Source: CAD feature listing. Evaluate the final solid. Frame: model axes, mm. A direction names the side the tool comes from. Give positions to 0.01 mm unless a question says otherwise; leave off trailing zeros. Loops run counter-clockwise (first coordinate to the right, second up) from the corner with the lowest first, then second, coordinate; pieces in that order, holes last. Notation, with made-up numbers: (16.25, -19.75) -> (52.25, -19.75) arc R17 cw to (52.25, 5.25) -> close; hole circle Ø8 at (12.25, -21). An arc over 180 degrees is marked (long way). Return JSON: item names as keys, results as strings. Group by question number.
(1) Ray query, line 1 (Z direction, x = 0, y = 85.15) (3 decimals); line 2 (Z direction, x = 0, y = 87.5) (3 decimals); line 3 (Y direction, x = 0, z = 28.7) (3 decimals). Return the intervals inside material, ascending. Write a range as from..to.
(2) Cut plane A-A on y = 74.7. Return loops of the section in (x, z), then the cut area to 3 significant figures.
(3) Draft query along Y for faces 1 (the face through (0.5, 61, 11)), 2 (the face through (0, 82, 13)), 3 (the face through (0, 63, 27.5)), 4 (the face through (4.5, 48, 17)). Return one class per face: released by +Y, released by -Y, zero draft, split by the parting line, or undercut.
(4) Cut plane C-C on z = 30.5. Return loops of the section in (x, y) (3 decimals), then the cut area to 3 significant figures.
(5) Cut plane D-D on y = 63. Return loops of the section in (x, z), then the cut area to 3 significant figures.
(6) Access query for faces 5 (the face through (0, 82, 21)), 6 (the face through (2.528, 64.794, 8.081)), 7 (the face through (-0.11, 6.764, 10.873)). Directions: +Z, -Z, +X, -X, +Y, -Y. A direction counts if a zero-diameter tool reaches every point of the face in a straight line with its end or side. Return the directions, or none.
(7) Cut plane B-B on z = 8. Return loops of the section in (x, y) (3 decimals), then the cut area to 3 significant figures.
(8) Pin query (flat end, axial travel): pin 1 (1.4 mm diameter, centred on x = 0, z = 12, fed in from +Y); pin 2 (3 mm diameter, centred on x = -0.5, z = 8, fed in from -Y); pin 3 (4 mm diameter, centred on x = -1, y = 41, fed in from -Z); pin 4 (2 mm diameter, centred on x = -0.5, y = 64, fed in from +Z). Return the tip coordinate at first contact, or that it passes through.
Autodesk Inventor part; units mm, degrees
ref_plane "Work Plane2" through (-89, -40.3889, 33.5) normal (0, 0, 1) x (1, 0, 0)
ref_plane "YZ Plane" through (0, 0, 0) normal (1, 0, 0) x (0, 1, 0)
ref_plane "XZ Plane" through (0, 0, 0) normal (0, 1, 0) x (-1, 0, 0)
ref_plane "Work Plane1" through (0, 0, 0) normal (0, 0, 1) x (1, 0, 0)
ref_plane "Work Plane2" through (-89, -40.3889, 33.5) normal (0, 0, 1) x (1, 0, 0)
sketch "Sketch1" plane through (0, 0, 0) normal (0, 0, 1) x (1, 0, 0)
  line L0 (23.5, 88.5) -> (-23.5, 88.5)
  line L1 (-23.5, 88.5) -> (-23.5, 36.5)
  line L2 (-26.5, 33.5) -> (-89, 33.5)
  line L3 (-89, 33.5) -> (-89, -72.5)
  line L4 (-89, -72.5) -> (-77, -72.5)
  line L5 (-74, -75.5) -> (-74, -93.5)
  line L6 (-74, -93.5) -> (74, -93.5)
  line L7 (74, -93.5) -> (74, -75.5)
  line L8 (77, -72.5) -> (89, -72.5)
  line L9 (89, -72.5) -> (89, 33.5)
  line L10 (89, 33.5) -> (26.5, 33.5)
  line L11 (23.5, 36.5) -> (23.5, 88.5)
  line L12 (-4.5, 81.5) -> (-4.5, 36.5)
  line L13 (-7.5, 33.5) -> (-13.5, 33.5)
  line L14 (-16.5, 36.5) -> (-16.5, 81.5)
  line L15 (7.5, 84.5) -> (13.5, 84.5)
  line L16 (16.5, 81.5) -> (16.5, 36.5)
  line L17 (13.5, 33.5) -> (7.5, 33.5)
  line L18 (4.5, 36.5) -> (4.5, 81.5)
  line L19 (-13.5, 84.5) -> (-7.5, 84.5)
  line L20 (-4.5, 88.5) -> (4.5, 88.5)
  line L21 (4.5, 88.5) -> (4.5, 5.75)
  line L22 (4.5, 5.75) -> (-4.5, 5.75)
  line L23 (-4.5, 5.75) -> (-4.5, 88.5)
  line L24 (-32.2, 4.75) -> (-59.9, 4.75)
  arc A0 (13.5, 33.5) -> (16.5, 36.5) centre (13.5, 36.5) ccw
  arc A1 (4.5, 36.5) -> (7.5, 33.5) centre (7.5, 36.5) ccw
  arc A2 (7.5, 84.5) -> (4.5, 81.5) centre (7.5, 81.5) ccw
  arc A3 (16.5, 81.5) -> (13.5, 84.5) centre (13.5, 81.5) ccw
  arc A4 (-4.5, 81.5) -> (-7.5, 84.5) centre (-7.5, 81.5) ccw
  arc A5 (-7.5, 33.5) -> (-4.5, 36.5) centre (-7.5, 36.5) ccw
  arc A6 (-16.5, 36.5) -> (-13.5, 33.5) centre (-13.5, 36.5) ccw
  arc A7 (-13.5, 84.5) -> (-16.5, 81.5) centre (-13.5, 81.5) ccw
  arc A8 (-26.5, 33.5) -> (-23.5, 36.5) centre (-26.5, 36.5) ccw
  arc A9 (-74, -75.5) -> (-77, -72.5) centre (-77, -75.5) ccw
  arc A10 (77, -72.5) -> (74, -75.5) centre (77, -75.5) ccw
  arc A11 (23.5, 36.5) -> (26.5, 33.5) centre (26.5, 36.5) ccw
  circle A12 centre (21.5, -85.5) radius 1.8
  circle A13 centre (-64.5, -85.5) radius 1.8
  circle A14 centre (83.4, -16.3889) radius 1.8
  circle A15 centre (-83.4, -19.2889) radius 1.8
  circle A16 centre (-21.5, -85.5) radius 1.8
  circle A17 centre (64.5, -85.5) radius 1.8
  circle A18 centre (-56.0375, 15.0937) radius 1.0065
  circle A19 centre (39.125, 4.3375) radius 1.0065
  circle A20 centre (-72.95, 4.275) radius 1.0065
  circle A21 centre (39.125, 25.9125) radius 1.0065
  circle A22 centre (72.95, 12.275) radius 1.0065
  circle A23 centre (86, 30.5) radius 1.0065
  circle A24 centre (-86, 30.5) radius 1.0065
  circle A25 centre (-39.125, 12.3375) radius 1.0065
  circle A26 centre (-72.95, 25.975) radius 1.0065
  circle A27 centre (-72.95, 12.275) radius 1.0065
  circle A28 centre (-39.125, 25.9125) radius 1.0065
  circle A29 centre (-86, 7.75) radius 1.0065
  circle A30 centre (86, 7.75) radius 1.0065
  circle A31 centre (72.95, 25.975) radius 1.0065
  circle A32 centre (39.125, 12.3375) radius 1.0065
  circle A33 centre (-39.125, 4.3375) radius 1.0065
  circle A34 centre (72.95, 4.275) radius 1.0065
  circle A35 centre (56.0375, 15.125) radius 1.0065
  circle A36 centre (78, -67.1725) radius 1.2295
  circle A37 centre (-24.1, -73.1) radius 1.2295
  circle A38 centre (24.1, -24.9) radius 1.2295
  circle A39 centre (-42.5, -43.2802) radius 1.2295
  circle A40 centre (-79, -42.3889) radius 1.2295
  circle A41 centre (-19.5, 28.875) radius 1.2295
  circle A42 centre (19.5, 9.55) radius 1.2295
  circle A43 centre (19.5, 47.3) radius 1.2295
  circle A44 centre (-19.5, 47.3) radius 1.2295
  circle A45 centre (0, 74.7) radius 1.2295
  circle A46 centre (-19.4231, 74.8077) radius 1.2295
  circle A47 centre (19.5, 74.7) radius 1.2295
  circle A48 centre (0, 49.05) radius 1.2295
  circle A49 centre (19.5, 28.875) radius 1.2295
  circle A50 centre (0, 19.125) radius 1.2295
  circle A51 centre (-19.5, 9.55) radius 1.2295
  circle A52 centre (-78, -67.1725) radius 1.2295
  circle A53 centre (-24.1, -24.9) radius 1.2295
  circle A54 centre (24.1, -73.1) radius 1.2295
  circle A55 centre (42.5, -42.7745) radius 1.2295
  circle A56 centre (79, -42.3889) radius 1.2295
  point P0 (0, 0)
  point P1 (-4.5, 81.5)
  point P2 (-4.5, 36.5)
  point P3 (7.5, 81.5)
  point P4 (13.5, 81.5)
  point P5 (-7.5, 81.5)
  point P6 (-13.5, 81.5)
  dimension "d41" = 1
extrude "Extrusion1" add sketch "Sketch1" along normal up to surface (33.5 mm away) contours L21 L18 L22 L23 L12 L0 | A45 | A48 | A50
sketch "Sketch2" plane through (4.5, 5.75, 0) normal (1, 0, 0) x (0, 0, -1)
  circle A0 centre (-23.4363, 28.1825) radius 2
  point P0 (0, -5.75)
extrude "Extrusion2" cut sketch "Sketch2" against normal blind 10
sketch "Sketch3" plane through (4.5, 5.75, 0) normal (1, 0, 0) x (0, 0, -1)
  circle A0 centre (-10.5, 55.25) radius 4.5
  point P0 (0, -5.75)
extrude "Extrusion3" cut sketch "Sketch3" against normal blind 4
sketch "Sketch4" plane through (-4.5, 5.75, 0) normal (-1, 0, 0) x (0, 0, 1)
  circle A0 centre (10.5, 55.25) radius 4.5
  point P0 (0, -5.75)
extrude "Extrusion4" cut sketch "Sketch4" against normal blind 4
sketch "Sketch5" plane through (-4.5, 5.75, 33.5) normal (0, 0, 1) x (1, 0, 0)
  line L0 (5, 59.75) -> (5, 50.75)
  line L1 (4, 50.75) -> (4, 59.75)
  line L2 (9, 26.1825) -> (0, 26.1825)
  line L3 (9, 30.1825) -> (0, 30.1825)
  line L4 (17, 78.15) -> (-8, 78.15)
  line L5 (-8, 35.85) -> (17, 35.85)
  line L6 (9, 82.75) -> (9, 0)
  line L7 (0, 50.75) -> (0, 59.75)
  line L8 (9, 35.85) -> (0, 35.85)
  line L9 (0, 35.85) -> (0, 50.75)
  line L10 (0, 50.75) -> (9, 50.75)
  line L11 (9, 50.75) -> (9, 35.85)
  line L12 (0, 0) -> (0, 82.75)
  line L13 (9, 78.15) -> (0, 78.15)
  line L14 (0, 78.15) -> (0, 59.75)
  line L15 (0, 59.75) -> (9, 59.75)
  line L16 (9, 59.75) -> (9, 78.15)
  line L17 (-18, 6.625) -> (-18, 20.125)
  line L18 (-18, 13.375) -> (27, 13.375)
  line L19 (9, 35.85) -> (0, 50.75)
  line L20 (9, 59.75) -> (9, 50.75)
  line L21 (0, 35.85) -> (9, 50.75)
  line L22 (9, 59.75) -> (0, 78.15)
  line L23 (0, 59.75) -> (9, 78.15)
  point P0 (4.5, -5.75)
  point P1 (4.5, 13.375)
  point P2 (4.5, 43.3)
  point P3 (4.5, 68.95)
  dimension "d9" = 4.5
  dimension "d10" = 4.5
hole "Hole1" at (0, 19.125, 33.5) at (0, 49.05, 33.5) at (0, 74.7, 33.5) direction (0, 0, -1) diameter 3.6 end through all countersink diameter 6.6 countersink angle 90
sketch "Sketch6" plane through (-4.5, 5.75, 0) normal (0, -1, 0) x (1, 0, 0)
  line L0 (9, 33.5) -> (0, 33.5)
  line L1 (0, 0) -> (0, 33.5)
  line L2 (0, 0) -> (9, 0)
  line L3 (9, 0) -> (9, 33.5)
  line L4 (0, 16.75) -> (9, 16.75)
  line L5 (9, 16.75) -> (0, 33.5)
  line L6 (9, 33.5) -> (0, 16.75)
  line L7 (0, 16.75) -> (9, 0)
  line L8 (9, 16.75) -> (0, 0)
  point P0 (4.5, 0)
  point P1 (4.5, 8.375)
  point P2 (4.5, 25.125)
hole "Hole2" at (0, 5.75, 8.375) at (0, 5.75, 25.125) direction (0, 1, 0) diameter 4 depth 6.6 counterbore diameter 5 counterbore depth 2
sketch "Sketch7" plane through (-4.5, 88.5, 0) normal (0, 1, 0) x (1, 0, 0)
  line L0 (0, -33.5) -> (9, -33.5)
  line L1 (0, -33.5) -> (9, -33.5)
  line L2 (9, 0) -> (9, -33.5)
  line L3 (9, 0) -> (0, 0)
  line L4 (0, 0) -> (0, -33.5)
  line L5 (-8, -1.4) -> (-8, -6.6)
  line L6 (-8, -32.1) -> (-8, -26.9)
  line L7 (17, -32.1) -> (17, -26.9)
  line L8 (17, -1.4) -> (17, -6.6)
  line L9 (17, -32.1) -> (-8, -32.1)
  line L10 (-8, -32.1) -> (-8, -26.9)
  line L11 (-8, -26.9) -> (17, -26.9)
  line L12 (17, -26.9) -> (17, -32.1)
  line L13 (-8, -6.6) -> (17, -6.6)
  line L14 (17, -6.6) -> (17, -1.4)
  line L15 (17, -1.4) -> (-8, -1.4)
  line L16 (-8, -1.4) -> (-8, -6.6)
  line L17 (17, -6.6) -> (-8, -6.6)
  line L18 (-8, -6.6) -> (-8, -8.6)
  line L19 (-8, -8.6) -> (17, -8.6)
  line L20 (17, -8.6) -> (17, -6.6)
  line L21 (-8, -26.9) -> (17, -26.9)
  line L22 (17, -26.9) -> (17, -24.9)
  line L23 (17, -24.9) -> (-8, -24.9)
  line L24 (-8, -24.9) -> (-8, -26.9)
  line L25 (9, 0) -> (9, -33.5)
  line L26 (9, -16.75) -> (0, -16.75)
  line L27 (0, 0) -> (0, -33.5)
  line L28 (9, -24.9) -> (0, -16.75)
  line L29 (9, -8.6) -> (0, -16.75)
  line L30 (0, -8.6) -> (9, -16.75)
  line L31 (9, -16.75) -> (0, -24.9)
  point P0 (4.5, 0)
  point P1 (4.5, -20.825)
  point P2 (4.5, -12.675)
  dimension "d25" = 2
  dimension "d26" = 2
hole "Hole3" at (0, 88.5, 20.825) at (0, 88.5, 12.675) direction (0, -1, 0) diameter 4 depth 6.5 counterbore diameter 4.6 counterbore depth 2
sketch "Sketch8" plane through (-4.5, 5.75, 33.5) normal (0, 0, 1) x (1, 0, 0)
  line L0 (26, 27.2497) -> (-17, 27.2497)
  line L1 (26, 31.2497) -> (-17, 31.2497)
  line L2 (4, 52.75) -> (-1, 52.75)
  line L3 (4, 61.75) -> (-1, 61.75)
  line L4 (10, 61.75) -> (5, 61.75)
  line L5 (9, 50.75) -> (5, 50.75)
  line L6 (0, 0) -> (0, 82.75)
  line L7 (9, 52.75) -> (0, 52.75)
  line L8 (0, 52.75) -> (0, 61.75)
  line L9 (0, 61.75) -> (9, 61.75)
  line L10 (9, 61.75) -> (9, 50.75)
  line L11 (9, 26.1825) -> (0, 26.1825)
  line L12 (0, 31.2497) -> (9, 31.2497)
  line L13 (9, 31.2497) -> (9, 26.1825)
  line L14 (9, 26.1825) -> (0, 26.1825)
  line L15 (0, 26.1825) -> (0, 31.2497)
  line L16 (9, 26.1825) -> (0, 31.2497)
  line L17 (0, 26.1825) -> (9, 31.2497)
  line L18 (10, 51.75) -> (0, 61.75)
  line L19 (0, 52.75) -> (9, 61.75)
  point P0 (4.5, -5.75)
  point P1 (4.5, 28.7161)
  point P2 (4.5, 57.25)
hole "Hole4" at (0, 34.4661, 33.5) at (0, 63, 33.5) direction (0, 0, -1) diameter 4 depth 6 counterbore diameter 4.6 counterbore depth 1.5
properties part number "middle_gear_holder" material "Nylon 6/6"
Answers:
{
 "1": {"line 1": "0..10.675, 14.675..18.825, 22.825..33.5", "line 2": "0..10.375, 14.975..18.525, 23.125..33.5", "line 3": "5.75..17.325, 20.925..32.466, 36.466..47.25, 50.85..61, 65..72.9, 76.5..88.5"},
 "2": {"outline": "(-4.5, 0) -> (-1.8, 0) -> (-1.8, 32) -> (-3.3, 33.5) -> (-4.5, 33.5) -> close; (1.8, 0) -> (4.5, 0) -> (4.5, 33.5) -> (3.3, 33.5) -> (1.8, 32) -> close", "area": "179 mm²"},
 "3": {"face 1": "undercut", "face 2": "released by +Y", "face 3": "undercut", "face 4": "zero draft"},
 "4": {"outline": "(-4.5, 5.75) -> (4.5, 5.75) -> (4.5, 88.5) -> (-4.5, 88.5) -> close; hole circle Ø4 at (0, 34.466); hole circle Ø4 at (0, 63); hole circle Ø3.6 at (0, 19.125); hole circle Ø3.6 at (0, 49.05); hole circle Ø3.6 at (0, 74.7)", "area": "689 mm²"},
 "5": {"outline": "(-4.5, 0) -> (4.5, 0) -> (4.5, 6.47) -> (0.5, 6.47) -> (0.5, 14.53) -> (4.5, 14.53) -> (4.5, 33.5) -> (2.3, 33.5) -> (2.3, 32) -> (2, 32) -> (2, 27.5) -> (-2, 27.5) -> (-2, 32) -> (-2.3, 32) -> (-2.3, 33.5) -> (-4.5, 33.5) -> (-4.5, 14.53) -> (-0.5, 14.53) -> (-0.5, 6.47) -> (-4.5, 6.47) -> close", "area": "212 mm²"},
 "6": {"face 5": "+Y", "face 6": "+X", "face 7": "-Y"},
 "7": {"outline": "(-4.5, 5.75) -> (-2.472, 5.75) -> (-2.472, 7.75) -> (-1.965, 7.75) -> (-1.965, 12.35) -> (1.965, 12.35) -> (1.965, 7.75) -> (2.472, 7.75) -> (2.472, 5.75) -> (4.5, 5.75) -> (4.5, 57.258) -> (0.5, 57.258) -> (0.5, 64.742) -> (4.5, 64.742) -> (4.5, 88.5) -> (-4.5, 88.5) -> (-4.5, 64.742) -> (-0.5, 64.742) -> (-0.5, 57.258) -> (-4.5, 57.258) -> close; hole circle Ø3.6 at (0, 19.125); hole circle Ø3.6 at (0, 49.05); hole circle Ø3.6 at (0, 74.7)", "area": "626 mm²"},
 "8": {"pin 1": "y = 82", "pin 2": "y = 7.75", "pin 3": "z = 0", "pin 4": "z = 32"}
}
